Here's how the part is built. I have some questions about the finished solid (model axes, mm). A direction names the side the tool comes from. Round coordinates to 2 decimals unless told otherwise and drop trailing zeros. Order: outer loops, then holes, each group sorted by start corner. A loop starts at its lowest first (then second) coordinate and runs counter-clockwise, first axis right, second up. Notation, with made-up numbers: M -5,4.5 L 29,4.5 A23 ccw 29,37.5 Z; hole C -7.75,-33 d1. An arc over 180 degrees is marked long. Write item = value, one per line. Start each with the question number.
Item 1: For faces 4 (the face through (5.901, 0.986, 61.752)), 5 (the face through (25, 48, 35)), which set-ups out of +Z, -Z, +X, -X, +Y, -Y let a thin tool reach every point of the face, with its end or its side?
Item 2: I want a section at A-A, the plane y = 18. List the corners of the cut face in (x, z) for me, plus the area to 3 significant figures.
Item 3: I want a section at D-D, the plane z = 64. List the corners of the cut face in (x, y) for me.
Item 4: I want a section at B-B, the plane z = 6. List the corners of the cut face in (x, y) for me, plus the area to 3 significant figures.
Item 5: Please list where these lines run through material, in increasing order: L1, parallel to Z at x = 6, y = 1; L2, parallel to X at y = 49.05, z = 64; L3, parallel to Y at x = 10, z = 7.5.
Item 6: I want a section at C-C, the plane x = 44. List the corners of the cut face in (y, z) for me, plus the area to 3 significant figures.
Item 7: We'd pull the mould along Y, two halves only. Please class faces 1 (the face through (25, 0, 35)), 2 (the face through (41.77, 0.99, 63.71)), 3 (the face through (25, 2, 35)): pulls with the +Y half, pulls with the -Y half, needs draft (parallel to the pull), parting line crosses it, or undercut.
Autodesk Inventor part; units mm, degrees
ref_plane "YZ Plane" through (0, 0, 0) normal (1, 0, 0) x (0, 1, 0)
ref_plane "XZ Plane" through (0, 0, 0) normal (0, 1, 0) x (-1, 0, 0)
ref_plane "XY Plane" through (0, 0, 0) normal (0, 0, 1) x (1, 0, 0)
sketch "スケッチ1" plane through (0, 0, 0) normal (0, 0, 1) x (1, 0, 0)
  line L0 (0, 0) -> (50, 0)
  line L1 (50, 0) -> (50, 50)
  line L2 (50, 50) -> (0, 50)
  line L3 (0, 50) -> (0, 0)
  line L4 (2, 48) -> (48, 48)
  line L5 (48, 48) -> (48, 2)
  line L6 (48, 2) -> (2, 2)
  line L7 (2, 2) -> (2, 48)
  dimension "d0" = 50
  dimension "d1" = 50
  dimension "d2" = 2
extrude "押し出し1" add sketch "スケッチ1" along normal blind 70
sketch "スケッチ2" plane through (0, 50, 0) normal (0, 1, 0) x (1, 0, 0)
  line L0 (50, 0) -> (0, 0)
  line L1 (0, 0) -> (0, -70)
  line L2 (50, -70) -> (0, -70)
  line L3 (50, 0) -> (50, -70)
  line L4 (50, -64) -> (0, -64) construction
  point P0 (0, 0)
  point P1 (44, -64)
  point P2 (6, -64)
  dimension "d6" = 6
  dimension "d7" = 38
  dimension "d24" = 6
hole "穴1" at (44, 50, 64) at (6, 50, 64) direction (0, -1, 0) diameter 4.5 end through all
sketch "スケッチ4" plane through (0, 50, 0) normal (0, 1, 0) x (1, 0, 0)
  circle A0 centre (44, -64) radius 2.25
  circle A1 centre (6, -64) radius 2.25
  line L0 (50, 0) -> (0, 0)
  line L1 (0, 0) -> (0, -70)
  line L2 (50, -70) -> (0, -70)
  line L3 (50, 0) -> (50, -70)
  line L4 (6, -70) -> (6, 0) construction
  point P0 (0, 0)
  point P1 (6, -6)
  point P2 (6, -44)
  dimension "d25" = 6
  dimension "d26" = 6
  dimension "d27" = 38
hole "穴3" at (6, 50, 6) at (6, 50, 44) direction (0, -1, 0) diameter 4.5 end through all
properties part number "hip" material "アルミニウム 6061"
Filled in:
q1.face_4 = +Y, -Y
q1.face_5 = +Z, -Z
q2.outline = M 0,0 L 2,0 L 2,70 L 0,70 Z; M 48,0 L 50,0 L 50,70 L 48,70 Z
q2.area = 280 mm^2
q3.outline = M 0,0 L 3.75,0 L 3.75,2 L 2,2 L 2,48 L 3.75,48 L 3.75,50 L 0,50 Z; M 8.25,0 L 41.75,0 L 41.75,2 L 8.25,2 Z; M 8.25,48 L 41.75,48 L 41.75,50 L 8.25,50 Z; M 46.25,0 L 50,0 L 50,50 L 46.25,50 L 46.25,48 L 48,48 L 48,2 L 46.25,2 Z
q4.outline = M 0,0 L 3.75,0 L 3.75,2 L 2,2 L 2,48 L 3.75,48 L 3.75,50 L 0,50 Z; M 8.25,0 L 50,0 L 50,50 L 8.25,50 L 8.25,48 L 48,48 L 48,2 L 8.25,2 Z
q4.area = 366 mm^2
q5.L1 = 0 to 3.75, 8.25 to 41.75, 46.25 to 61.75, 66.25 to 70
q5.L2 = 0 to 3.75, 8.25 to 41.75, 46.25 to 50
q5.L3 = 0 to 2, 48 to 50
q6.outline = M 0,0 L 2,0 L 2,61.75 L 0,61.75 Z; M 0,66.25 L 2,66.25 L 2,70 L 0,70 Z; M 48,0 L 50,0 L 50,61.75 L 48,61.75 Z; M 48,66.25 L 50,66.25 L 50,70 L 48,70 Z
q6.area = 262 mm^2
q7.face_1 = pulls with the -Y half
q7.face_2 = needs draft
q7.face_3 = undercut
